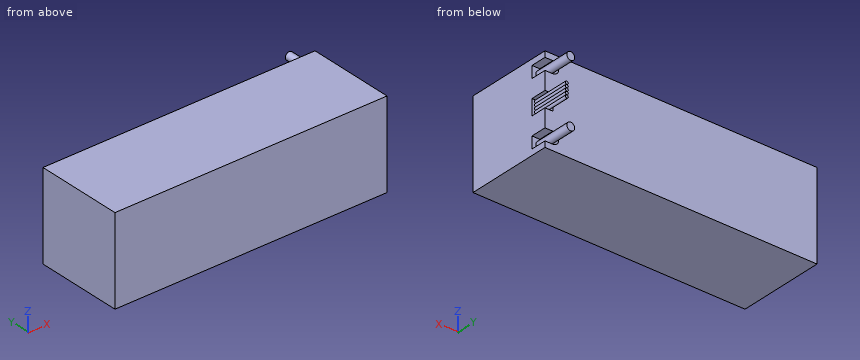
from build123d import *

# Parameters (mm, degrees)
SKETCH1_W           = 138.90625
SKETCH1_H           = 44.45
BOSS_EXTRUDE1_DEPTH = 44.45
SKETCH2_W           = 4
SKETCH2_H           = 8
CUT_EXTRUDE1_DEPTH  = 8
SKETCH3_R           = 2
SKETCH3_R_2         = 0.75
BOSS_EXTRUDE2_DEPTH = 19.05


with BuildPart() as part:
    # Sketch1 → Boss-Extrude1 (new body)
    with BuildSketch(Plane.XY):
        Rectangle(SKETCH1_W, SKETCH1_H)
    extrude(amount=BOSS_EXTRUDE1_DEPTH)

    # Sketch2 → Cut-Extrude1 (cut)
    with BuildSketch(Plane(origin=(0, 22.225, 0), x_dir=(1, 0, 0), z_dir=(0, 1, 0))):
        with BuildLine():
            Line((65.453125, -35.45), (69.453125, -35.45))
            Line((69.453125, -35.45), (69.453125, -41.45))
            Line((69.453125, -41.45), (65.453125, -41.45))
            ThreePointArc((65.453125, -41.45), (62.453125, -38.45), (65.453125, -35.45))
        make_face()
        with BuildLine():
            Line((69.453125, -3), (65.453125, -3))
            ThreePointArc((65.453125, -3), (62.453125, -6), (65.453125, -9))
            Line((65.453125, -9), (69.453125, -9))
            Line((69.453125, -9), (69.453125, -3))
        make_face()
        with Locations((67.453125, -22.225)):
            Rectangle(SKETCH2_W, SKETCH2_H)
    extrude(amount=-CUT_EXTRUDE1_DEPTH, mode=Mode.SUBTRACT)

    # Sketch3 → Boss-Extrude2 (add)
    with BuildSketch(Plane(origin=(0, 14.225, 0), x_dir=(1, 0, 0), z_dir=(0, 1, 0))):
        with Locations((65.453125, -38.45)):
            Circle(SKETCH3_R)
        with Locations((65.453125, -6)):
            Circle(SKETCH3_R)
        with Locations((67.453125, -19.0241)):
            Circle(SKETCH3_R_2)
        with Locations((67.453125, -20.6243)):
            Circle(SKETCH3_R_2)
        with Locations((67.453125, -22.2245)):
            Circle(SKETCH3_R_2)
        with Locations((67.453125, -23.8247)):
            Circle(SKETCH3_R_2)
        with Locations((67.453125, -25.4249)):
            Circle(SKETCH3_R_2)
    extrude(amount=BOSS_EXTRUDE2_DEPTH)


solid = part.part
Geometry: final body of the model. Coordinates: model frame, mm. Round coordinates to 2 decimals unless told otherwise and drop trailing zeros. Loops run counter-clockwise (first coordinate to the right, second up) from the corner with the lowest first, then second, coordinate; pieces in that order, holes last. Notation, with made-up numbers: (-36, -3.75) - (-7, -3.75) arc R13 ccw to (-7, 6.25) - close; hole circle Ø7 at (68, -37). An arc over 180 degrees is marked (long way). Write each question's results on one line, items separated by ' | '. Start each with the question number.
1) Cut plane B-B on y = 27.5. Return loops of the section in (x, z), then the cut area to 3 significant figures.
2) Cut plane A-A on z = 38.45. Return loops of the section in (x, y) (3 decimals), then the cut area to 3 significant figures.
3) First-contact query: P1, Ø4, axis at x = -47, z = 34.5, coming from the +Y side (3 decimals); P2, Ø4, axis at y = 18, z = 22.5, coming from the +X side. Flat tips, straight axial feed; report the tip coordinate or a pass-through.
4) Line query: probe 1 along Y at (x, z) = (31, 41.5) (3 decimals); probe 2 along X at (y, z) = (25.5, 6); probe 3 along X at (y, z) = (14.5, 21). Output: solid intervals per line, ascending. Write a range as [from, to].
5) Cut plane C-C on x = -15. Return loops of the section in (y, z) (3 decimals).
Verdict:
1) outline: circle Ø4 at (65.45, 6); circle Ø4 at (65.45, 38.45); circle Ø1.5 at (67.45, 19.02); circle Ø1.5 at (67.45, 20.62); circle Ø1.5 at (67.45, 22.22); circle Ø1.5 at (67.45, 23.82); circle Ø1.5 at (67.45, 25.42) | area: 34.0 mm2
2) outline: (-69.453, -22.225) - (69.453, -22.225) - (69.453, 14.225) - (67.453, 14.225) - (67.453, 33.275) - (63.453, 33.275) - (63.453, 14.225) - (62.453, 14.225) - (62.453, 22.225) - (-69.453, 22.225) - close | area: 6,190 mm2
3) P1: stops at y = 22.225 | P2: stops at x = 68.2
4) probe 1: y = [-22.225, 22.225] | probe 2: x = [63.45, 67.45] | probe 3: x = [-69.45, 65.45], [66.8, 68.1]
5) outline: (-22.225, 0) - (22.225, 0) - (22.225, 44.45) - (-22.225, 44.45) - close
